Autodesk Inventor part; units mm, degrees
ref_plane "YZ Plane" through (0, 0, 0) normal (1, 0, 0) x (0, 1, 0)
ref_plane "XZ Plane" through (0, 0, 0) normal (0, 1, 0) x (-1, 0, 0)
ref_plane "XY Plane" through (0, 0, 0) normal (0, 0, 1) x (1, 0, 0)
sketch "Sketch1" plane through (0, 0, 0) normal (0, 1, 0) x (-1, 0, 0)
  line L0 (-29.02, 49.29) -> (29.02, 49.29)
  line L1 (29.02, 49.29) -> (29.02, 40.715) construction
  line L2 (29.02, -49.29) -> (-29.02, -49.29)
  line L3 (-29.02, -49.29) -> (-29.02, -40.715) construction
  line L4 (-29.02, 49.29) -> (29.02, -49.29) construction
  line L5 (29.02, 49.29) -> (-29.02, -49.29) construction
  line L6 (-33, 45) -> (33, 45) construction
  line L7 (33, 45) -> (33, -45) construction
  line L8 (33, -45) -> (-33, -45) construction
  line L9 (-33, -45) -> (-33, 45) construction
  line L10 (-33, 45) -> (33, -45) construction
  line L11 (33, 45) -> (-33, -45) construction
  circle A0 centre (33, 45) radius 1.5
  circle A1 centre (33, -45) radius 1.5
  circle A2 centre (-33, -45) radius 1.5
  circle A3 centre (-33, 45) radius 1.5
  line L12 (-38.27, 49.29) -> (38.27, 49.29) construction
  line L13 (38.27, 49.29) -> (38.27, -49.29) construction
  line L14 (38.27, -49.29) -> (-38.27, -49.29) construction
  line L15 (-38.27, -49.29) -> (-38.27, 49.29) construction
  line L16 (-38.27, 49.29) -> (38.27, -49.29) construction
  line L17 (38.27, 49.29) -> (-38.27, -49.29) construction
  line L18 (-38.27, 40.715) -> (29.02, 40.715) construction
  line L19 (38.27, 40.715) -> (38.27, -40.715) construction
  line L20 (38.27, -40.715) -> (-38.27, -40.715) construction
  line L21 (-38.27, -40.715) -> (-38.27, 40.715) construction
  line L22 (-38.27, 40.715) -> (38.27, -40.715) construction
  line L23 (38.27, 40.715) -> (-38.27, -40.715) construction
  line L24 (29.02, 49.29) -> (36.02, 49.29)
  line L25 (29.02, 40.715) -> (36.02, 40.715)
  arc A4 (36.02, 40.715) -> (36.02, 49.29) centre (33.06, 45.0025) ccw
  line L26 (29.02, 40.715) -> (29.02, -40.715)
  line L27 (0, 49.29) -> (0, -49.29) construction
  line L28 (-29.02, 0) -> (29.02, 0) construction
  line L29 (-38.27, -49.29) -> (38.27, -49.29) construction
  line L30 (-38.27, -40.715) -> (38.27, -40.715) construction
  line L31 (29.02, -49.29) -> (36.02, -49.29)
  line L32 (29.02, -40.715) -> (36.02, -40.715)
  arc A5 (36.02, -49.29) -> (36.02, -40.715) centre (33.06, -45.0025) ccw
  line L33 (0, -49.29) -> (0, 49.29) construction
  line L34 (-33, 45) -> (-33, -45) construction
  line L35 (38.27, 49.29) -> (-38.27, 49.29) construction
  line L36 (-38.27, 49.29) -> (-38.27, -49.29) construction
  line L37 (-38.27, -49.29) -> (38.27, -49.29) construction
  line L38 (38.27, 40.715) -> (-38.27, 40.715) construction
  line L39 (-38.27, -40.715) -> (38.27, -40.715) construction
  line L40 (-29.02, 49.29) -> (-36.02, 49.29)
  line L41 (-29.02, 40.715) -> (-36.02, 40.715)
  arc A6 (-36.02, 49.29) -> (-36.02, 40.715) centre (-33.06, 45.0025) ccw
  line L42 (38.27, -49.29) -> (-38.27, -49.29) construction
  line L43 (-29.02, -49.29) -> (-36.02, -49.29)
  line L44 (38.27, -40.715) -> (-38.27, -40.715) construction
  line L45 (-29.02, -40.715) -> (-36.02, -40.715)
  arc A7 (-36.02, -40.715) -> (-36.02, -49.29) centre (-33.06, -45.0025) ccw
  line L46 (-29.02, -40.715) -> (-29.02, 40.715)
  line L47 (-29.02, 40.715) -> (-29.02, 49.29) construction
  line L48 (29.02, 40.715) -> (38.27, 40.715) construction
  line L49 (29.02, -40.715) -> (29.02, -49.29) construction
  point P0 (0, 0)
  dimension "d0" = 58.04
  dimension "d1" = 98.58
  dimension "d2" = 66
  dimension "d3" = 90
  dimension "d4" = 3
  dimension "d5" = 3
  dimension "d6" = 3
  dimension "d7" = 3
  dimension "d8" = 76.54
  dimension "d9" = 98.58
  dimension "d10" = 76.54
  dimension "d11" = 81.43
  dimension "d12" = 7
  dimension "d13" = 7
extrude "Extrusion1" add sketch "Sketch1" along normal blind 2
sketch "Sketch2" plane through (0, 2, 0) normal (0, 1, 0) x (1, 0, 0)
  line L0 (29.02, -49.29) -> (-29.02, -49.29) construction
  line L1 (-29.02, -49.29) -> (-29.02, 49.29) construction
  line L2 (-29.02, 49.29) -> (29.02, 49.29) construction
  line L3 (29.02, 49.29) -> (29.02, -49.29) construction
  line L4 (29.02, -49.29) -> (-29.02, 49.29) construction
  line L5 (-29.02, -49.29) -> (29.02, 49.29) construction
  line L6 (29.02, 40.715) -> (29.02, -40.715)
  line L7 (-29.02, 49.29) -> (29.02, 49.29)
  line L8 (29.02, 49.29) -> (29.02, -40.71)
  line L9 (29.02, -40.71) -> (-29.02, -40.71)
  line L10 (-29.02, -40.71) -> (-29.02, 49.29)
  point P0 (0, 0)
  dimension "d16" = 58.04
  dimension "d17" = 98.58
  dimension "d18" = 90
extrude "Extrusion2" add sketch "Sketch2" along normal blind 18
sketch "Sketch3" plane through (-29.02, 0, -40.715) normal (-1, 0, 0) x (0, 0, 1)
  line L0 (-8.575, 0) -> (-8.575, 2)
  line L1 (-8.575, 0) -> (37.425, 0) construction
  line L2 (81.43, 0) -> (0, 0) construction
  line L3 (37.425, 0) -> (52.425, 0) construction
  line L4 (37.425, 0) -> (52.425, 0)
  line L5 (52.425, 0) -> (52.425, 20)
  line L6 (52.425, 20) -> (37.425, 20)
  line L7 (37.425, 20) -> (37.425, 0)
  line L8 (81.43, 0) -> (90.005, 0) construction
  line L9 (90.005, 0) -> (70.005, 0) construction
  line L10 (70.005, 0) -> (62.005, 0) construction
  line L11 (62.005, 0) -> (70.005, 0)
  line L12 (70.005, 0) -> (70.005, 20)
  line L13 (70.005, 20) -> (62.005, 20)
  line L14 (62.005, 20) -> (62.005, 0)
  point P0 (40.715, 0)
  dimension "d21" = 46
  dimension "d22" = 15
  dimension "d23" = 20
  dimension "d24" = 15
  dimension "d25" = 20
  dimension "d26" = 8
  dimension "d27" = 8
  dimension "d28" = 20
extrude "Extrusion3" add sketch "Sketch3" along normal blind 5
sketch "Sketch5" plane through (0, 0, 0) normal (0, -1, 0) x (1, 0, 0)
  circle A0 centre (-33, 45) radius 1.5 construction
  line L0 (33, -45) -> (-33, -45) construction
  line L1 (-33, -45) -> (-33, 45) construction
  line L2 (-33, 45) -> (33, 45) construction
  line L3 (33, 45) -> (33, -45) construction
  line L4 (33, -45) -> (-33, 45) construction
  line L5 (-33, -45) -> (33, 45) construction
  circle A1 centre (-33, -45) radius 1.5
  circle A2 centre (33, -45) radius 1.5
  circle A3 centre (33, 45) radius 1.5
  circle A4 centre (33, 45) radius 1.5
  circle A5 centre (-33, 45) radius 1.5
  line L6 (-35.5, -43.5566) -> (-33, -42.1132)
  line L7 (-33, -42.1132) -> (-30.5, -43.5566)
  line L8 (-30.5, -43.5566) -> (-30.5, -46.4434)
  line L9 (-30.5, -46.4434) -> (-33, -47.8868)
  line L10 (-33, -47.8868) -> (-35.5, -46.4434)
  line L11 (-35.5, -46.4434) -> (-35.5, -43.5566)
  line L12 (30.5, -43.5566) -> (33, -42.1132)
  line L13 (33, -42.1132) -> (35.5, -43.5566)
  line L14 (35.5, -43.5566) -> (35.5, -46.4434)
  line L15 (35.5, -46.4434) -> (33, -47.8868)
  line L16 (33, -47.8868) -> (30.5, -46.4434)
  line L17 (30.5, -46.4434) -> (30.5, -43.5566)
  line L18 (30.5, 46.4434) -> (33, 47.8868)
  line L19 (33, 47.8868) -> (35.5, 46.4434)
  line L20 (35.5, 46.4434) -> (35.5, 43.5566)
  line L21 (35.5, 43.5566) -> (33, 42.1132)
  line L22 (33, 42.1132) -> (30.5, 43.5566)
  line L23 (30.5, 43.5566) -> (30.5, 46.4434)
  line L24 (-35.5, 46.4434) -> (-33, 47.8868)
  line L25 (-33, 47.8868) -> (-30.5, 46.4434)
  line L26 (-30.5, 46.4434) -> (-30.5, 43.5566)
  line L27 (-30.5, 43.5566) -> (-33, 42.1132)
  line L28 (-33, 42.1132) -> (-35.5, 43.5566)
  line L29 (-35.5, 43.5566) -> (-35.5, 46.4434)
  point P0 (0, 0)
  point P1 (30.5, 45)
  point P2 (-35.5, 45)
  dimension "d31" = 3
  dimension "d32" = 3
  dimension "d33" = 3
  dimension "d34" = 3
  dimension "d35" = 5
  dimension "d36" = 5
  dimension "d37" = 5
  dimension "d38" = 5
extrude "Extrusion4" add sketch "Sketch5" against normal blind 22 from surface at -2
sketch "Sketch6" plane through (0, 0, 0) normal (0, -1, 0) x (1, 0, 0)
  line L0 (-35.8509, -30.6551) -> (-35.8509, -21.9955) construction
  line L1 (-35.8509, -21.9955) -> (-14.7214, -21.9955) construction
  line L2 (-14.7214, -21.9955) -> (-14.7214, -30.6551) construction
  line L3 (-14.7214, -30.6551) -> (-35.8509, -30.6551) construction
  point P0 (0, 0)
sketch "Sketch7" plane through (36.02, 0, -49.29) normal (0, 0, -1) x (-1, 0, 0)
  line L0 (36.02, 0) -> (63.02, 0) construction
  line L1 (0, 0) -> (72.04, 0)
  line L2 (63.02, 0) -> (11.02, 0)
  line L3 (11.02, 0) -> (11.02, 16)
  line L4 (11.02, 16) -> (63.02, 16)
  line L5 (63.02, 16) -> (63.02, 0)
  dimension "d41" = 27
  dimension "d42" = 52
  dimension "d43" = 16
extrude "Extrusion5" add sketch "Sketch7" along normal blind 2
sketch "Sketch8" plane through (0, 0, 0) normal (0, -1, 0) x (1, 0, 0)
  line L0 (-24.9386, -43.252) -> (-24.9386, 42.092) construction
  line L1 (-24.9386, 42.092) -> (23.0674, 42.092) construction
  line L2 (23.0674, 42.092) -> (23.0674, -43.252) construction
  line L3 (23.0674, -43.252) -> (-24.9386, -43.252) construction
  point P0 (0, 0)
equation "\"d24\" = d22"
properties part number "raspberry+touch"
The model under review builds one solid part; all positions refer to its coordinate system, in mm. A direction names the side the tool comes from. Round coordinates to 2 decimals unless told otherwise and drop trailing zeros. Order: outer loops, then holes, each group sorted by start corner. A loop starts at its lowest first (then second) coordinate and runs counter-clockwise, first axis right, second up.
(1) Take a section at C-C, the plane z = 45. State the section outline as (x, y) points.
Working result:
outline: (-38.27, 0) - (-34.5, 0) - (-34.5, 24) - (-35.5, 24) - (-35.5, 2) - (-38.27, 2) - close; (-31.5, 0) - (31.5, 0) - (31.5, 24) - (30.5, 24) - (30.5, 2) - (-30.5, 2) - (-30.5, 24) - (-31.5, 24) - close; (34.5, 0) - (38.27, 0) - (38.27, 2) - (35.5, 2) - (35.5, 24) - (34.5, 24) - close
(2) Mouldability with a two-part tool opening along X and no side actions: class faces 5 (the face through (-31, 10, 11.71)), 6 (the face through (30.5, 13, -45)), 7 (the face through (34.267, 12.846, 42.845)), 8 (the face through (31.733, 12.846, -42.845)) as released by +X, released by -X, zero draft, split by the parting line, or undercut.
Working result:
face 5: zero draft
face 6: undercut
face 7: released by +X
face 8: undercut
(3) Tool access review of faces 1 (the face through (34.267, 12.846, -47.155)), 2 (the face through (-35.5, 13, -45)), 3 (the face through (31.733, 12.846, 47.155)), 4 (the face through (0, 11, 40.71)): name each direction out of +Z, -Z, +X, -X, +Y, -Y from which nothing blocks a thin tool from reaching the whole face with its end or side.
Working result:
face 1: -Z, +X, +Y
face 2: +Z, -Z, -X, +Y
face 3: +Z, +Y
face 4: +Z, +X, -X, +Y
(4) Take a section at B-B, the plane x = -2. State the section outline as (y, z) points, plus the area to 3 significant figures.
Working result:
outline: (0, -51.29) - (16, -51.29) - (16, -49.29) - (20, -49.29) - (20, 40.71) - (2, 40.71) - (2, 49.29) - (0, 49.29) - close
area: 1,850 mm2
(5) Take a section at A-A, the plane z = -45. State the section outline as (x, y) points, plus the area to 3 significant figures.
Working result:
outline: (-38.27, 0) - (-34.5, 0) - (-34.5, 24) - (-35.5, 24) - (-35.5, 2) - (-38.27, 2) - close; (-31.5, 0) - (31.5, 0) - (31.5, 24) - (30.5, 24) - (30.5, 2) - (29.02, 2) - (29.02, 20) - (-29.02, 20) - (-29.02, 2) - (-30.5, 2) - (-30.5, 24) - (-31.5, 24) - close; (34.5, 0) - (38.27, 0) - (38.27, 2) - (35.5, 2) - (35.5, 24) - (34.5, 24) - close
area: 1,270 mm2
(6) For P1, Ø12, axis at x = -9, z = -38, coming from the +Y side; P2, Ø10, axis at y = 14.5, z = 22, coming from the -X side; P3, Ø1.4, axis at y = 8, z = -45, coming from the +X side, all flat-tipped, find the tip position at first contact; note any pin that passes through.
Working result:
P1: stops at y = 20
P2: stops at x = -34.02
P3: stops at x = 35.5
(7) Wall thickness on L1, parallel to X at y = 8.75, z = -45; L2, parallel to Z at x = -33, y = 12.75; L3, parallel to Z at x = 33, y = 1.45 (3 decimals): over which ranges is each line inside the solid? List them lowest first.
Working result:
L1: x = -35.5 to -34.5, -31.5 to -30.5, -29.02 to 29.02, 30.5 to 31.5, 34.5 to 35.5
L2: z = -47.89 to -46.5, -43.5 to -42.11, -3.29 to 11.71, 21.29 to 29.29, 42.11 to 43.5, 46.5 to 47.89
L3: z = -49.29 to -46.5, -43.5 to -40.715, 40.715 to 43.5, 46.5 to 49.29
(8) Take a section at D-D, the plane x = 27. State the section outline as (y, z) points, plus the area to 3 significant figures.
Working result:
outline: (0, -49.29) - (20, -49.29) - (20, 40.71) - (2, 40.71) - (2, 49.29) - (0, 49.29) - close
area: 1,820 mm2
